Part model, mm, in its own coordinate system. A direction names the side the tool comes from. Coordinates: 2 decimals unless noted, no trailing zeros. Write each loop counter-clockwise with the first axis right and the second up, starting at its lowest first coordinate (ties: lowest second). Pieces come first, ordered by that corner, then holes. Notation, with made-up numbers: (41.25, 12) - (89.25, 12) arc R24 ccw to (89.25, 26) - close; hole circle Ø5 at (-4.5, 6). An arc over 180 degrees is marked (long way). Use a Markdown table: item, result.
```python
from build123d import *

# Parameters (mm, degrees)
SKETCH1_W               = 25
SKETCH1_H               = 47.625
SKETCH1_R               = 2.6162
BOSS_EXTRUDE1_DEPTH     = 6
SKETCH3_W               = 52.5
SKETCH3_H               = 47.625
BOSS_EXTRUDE2_DEPTH     = 4
BOSS_EXTRUDE3_DEPTH     = 3
CUT_EXTRUDE1_DEPTH      = 72.101270207
CUT_EXTRUDE1_DEPTH_BACK = 72.101270207
SKETCH5_W               = 25
SKETCH5_H               = 4
CHAMFER1_SIZE           = 2
SKETCH6_W               = 6
SKETCH6_H               = 6.35
CUT_EXTRUDE2_DEPTH      = 74.928280279
CUT_EXTRUDE3_DEPTH      = 74.928280279
FILLET2_R               = 3
FILLET1_R               = 3
FILLET3_R               = 4


with BuildPart() as part:
    # Sketch1 → Boss-Extrude1 (new body)
    with BuildSketch(Plane.XY):
        with Locations((-12.5, -23.8125)):
            Rectangle(SKETCH1_W, SKETCH1_H)
        with Locations((-16, -11.1125)):
            Circle(SKETCH1_R, mode=Mode.SUBTRACT)
        with Locations((-16, -36.5125)):
            Circle(SKETCH1_R, mode=Mode.SUBTRACT)
    extrude(amount=-BOSS_EXTRUDE1_DEPTH)

    # Sketch3 → Boss-Extrude2 (add)
    with BuildSketch(Plane(origin=(0, 0, 0), x_dir=(0, 0, -1), z_dir=(1, 0, 0))):
        with Locations((26.25, -23.8125)):
            Rectangle(SKETCH3_W, SKETCH3_H)
    extrude(amount=-BOSS_EXTRUDE2_DEPTH)

    # Sketch4 → Boss-Extrude3 (add)
    with BuildSketch(Plane.XZ.offset(47.625)):
        Polygon((-25, -6), (-4, -52.5), (-4, -6), align=None)
    extrude(amount=-BOSS_EXTRUDE3_DEPTH)

    # Sketch5 → Cut-Extrude1 (cut, two sides: drawn at the far end of the back side and taken through both)
    with BuildSketch(Plane(origin=(0, 0, -6), x_dir=(-1, 0, 0), z_dir=(0, 0, -1)).offset(-CUT_EXTRUDE1_DEPTH_BACK)):
        with Locations((12.5, -2)):
            Rectangle(SKETCH5_W, SKETCH5_H)
    extrude(amount=CUT_EXTRUDE1_DEPTH + CUT_EXTRUDE1_DEPTH_BACK, mode=Mode.SUBTRACT)

    # Chamfer1
    chamfer1_edges = [part.edges().sort_by_distance(p)[0] for p in [
        (-14.5, -4, -6),
    ]]
    chamfer(chamfer1_edges, length=CHAMFER1_SIZE)

    # Sketch6 → Cut-Extrude2 (cut, through all)
    with BuildSketch(Plane.ZY.offset(4)):
        with Locations((-49.5, -20.701)):
            Rectangle(SKETCH6_W, SKETCH6_H)
    extrude(amount=-CUT_EXTRUDE2_DEPTH, mode=Mode.SUBTRACT)

    # Sketch7 → Cut-Extrude3 (cut, through all)
    with BuildSketch(Plane.ZY.offset(4)):
        with BuildLine():
            Line((-50.5, -4), (-6, -4))
            ThreePointArc((-6, -4), (-28.25, -9), (-50.5, -4))
        make_face()
    extrude(amount=-CUT_EXTRUDE3_DEPTH, mode=Mode.SUBTRACT)

    # Fillet2
    fillet2_edges = [part.edges().sort_by_distance(p)[0] for p in [
        (-2, -17.526, -46.5),
        (-2, -23.876, -46.5),
    ]]
    fillet(fillet2_edges, radius=FILLET2_R)
    fillet2_2_edges = [part.edges().sort_by_distance(p)[0] for p in [
        (-2, -17.526, -52.5),
        (-2, -23.876, -52.5),
    ]]
    fillet(fillet2_2_edges, radius=FILLET2_R - 0.0001)  # a hair under: the kernel refuses the full size

    # Fillet1
    fillet1_edges = [part.edges().sort_by_distance(p)[0] for p in [
        (-4, -25.3125, -6),
    ]]
    fillet(fillet1_edges, radius=FILLET1_R)

    # Fillet3
    fillet3_edges = [part.edges().sort_by_distance(p)[0] for p in [
        (-25, -4, -2),
    ]]
    fillet(fillet3_edges, radius=FILLET3_R)


solid = part.part
```
Item 1: Band-saw the part on B-B, the plane y = -29. Give the cut face in (x, z).
From the geometry:
| item | result |
|---|---|
| outline | (-25, -6) - (-7, -6) arc R3 cw to (-4, -9) - (-4, -52.5) - (0, -52.5) - (0, 0) - (-25, 0) - close |
Item 2: Drill centre lines: probe 1 along Y at (x, z) = (-16, -1.6) (3 decimals); probe 2 along Y at (x, z) = (-16, -4.1) (3 decimals); probe 3 along Y at (x, z) = (-16, -20) (3 decimals). Where is each one in solid material? Low to high.
From the geometry:
| item | result |
|---|---|
| probe 1 | -47.625 to -39.129, -33.896 to -13.729, -8.496 to -4 |
| probe 2 | -47.625 to -39.129, -33.896 to -13.729, -8.496 to -4.1 |
| probe 3 | -47.625 to -44.625 |
Item 3: Drop flat-ended pins along their axis: P1, Ø20.5, axis at y = -21.5, z = -31, coming from the -X side; P2, Ø10, axis at x = -20.5, y = -11, coming from the -Z side; P3, Ø1, axis at x = -4, z = -21, coming from the +Y side. Give the stop position or say it passes through.
From the geometry:
| item | result |
|---|---|
| P1 | x = -4 |
| P2 | z = -6 |
| P3 | y = -8.42 |
Item 4: Which spindle directions (+Z, -Z, +X, -X, +Y, -Y) get a long thin tool onto all of the face, cutting with end or side? Do faces 4 (the face through (-14, -5, -5)), 5 (the face through (-1.972, -24.731, -51.598)), 6 (the face through (-2, -9, -28)). Say none if no direction does.
From the geometry:
| item | result |
|---|---|
| face 4 | -Z, -X, +Y |
| face 5 | -Z, +X, -X |
| face 6 | +X, -X, +Y |
Item 5: Band-saw the part on A-A, the plane x = -16. Give the cut face in (y, z) (3 decimals).
From the geometry:
| item | result |
|---|---|
| outline | (-47.625, -25.929) - (-44.625, -25.929) - (-44.625, -6) - (-39.129, -6) - (-39.129, 0) - (-47.625, 0) - close; (-33.896, -6) - (-13.729, -6) - (-13.729, 0) - (-33.896, 0) - close; (-8.496, -6) - (-6, -6) - (-4, -4) - (-4, 0) - (-8.496, 0) - close |
Item 6: Band-saw the part on C-C, the plane x = -10.5. Give the cut face in (y, z) (3 decimals), then the cut area to 3 significant figures.
From the geometry:
| item | result |
|---|---|
| outline | (-47.625, -38.107) - (-44.625, -38.107) - (-44.625, -6) - (-6, -6) - (-4, -4) - (-4, 0) - (-47.625, 0) - close |
| area | 356 mm^2 |
Item 7: Two-plate mould, pull along Y, no slides. Class faces 1 (the face through (-16, -25, -6)), 2 (the face through (-1.972, -18.381, -47.402)), 3 (the face through (-23.859, -5.203, -2.375)): pulls with the +Y half, pulls with the -Y half, needs draft (parallel to the pull), parting line crosses it, or undercut.
From the geometry:
| item | result |
|---|---|
| face 1 | needs draft |
| face 2 | undercut |
| face 3 | pulls with the +Y half |
Item 8: Band-saw the part on D-D, the plane z = -45. Give the cut face in (x, y) (3 decimals), then the cut area to 3 significant figures.
From the geometry:
| item | result |
|---|---|
| outline | (-7.387, -47.625) - (0, -47.625) - (0, -6.229) - (-4, -6.229) - (-4, -44.625) - (-7.387, -44.625) - close |
| area | 176 mm^2 |
